The listing builds one solid part. Answer for the finished solid, in the listing's coordinates (mm). Give positions to 0.01 mm unless a question says otherwise; leave off trailing zeros. Write each loop counter-clockwise with the first axis right and the second up, starting at its lowest first coordinate (ties: lowest second). Pieces come first, ordered by that corner, then holes.
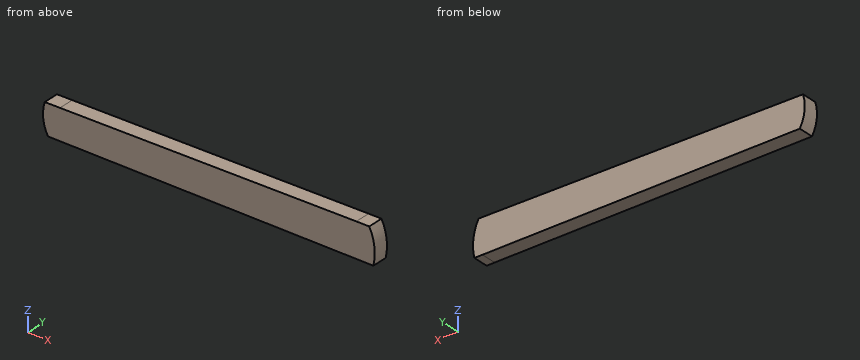
```python
from build123d import *

# Parameters (mm, degrees)
F2_DEPTH = 25


with BuildPart() as f2:
    # F1 (on face) → F2 (new body)
    with BuildSketch(Plane.XZ):
        with BuildLine():
            ThreePointArc((307.522314, 136.204265), (309.150117, 164.161267), (300.922203, 190.929627))
            Line((300.922203, 190.929627), (299.40453, 190.929627))
            Line((299.40453, 190.929627), (280.23421, 190.929627))
            Line((280.23421, 190.929627), (-194.487512, 188.015388))
            Line((-194.487512, 188.015388), (-218.880566, 187.865643))
            ThreePointArc((-218.880566, 187.865643), (-221.348908, 163.277257), (-213.697833, 139.779545))
            Line((-213.697833, 139.779545), (294.608427, 136.292847))
            Line((294.608427, 136.292847), (307.522314, 136.204265))
        make_face()
    extrude(amount=F2_DEPTH)


solid = f2.part
```
Item 1: Each of these flat-tipped pins is pushed along its axis until it touches: P1, Ø1, axis at y = -11, z = 149, coming from the -X side; P2, Ø4, axis at y = -14, z = 167, coming from the -X side; P3, Ø1.5, axis at x = 38.5, y = -3.5, coming from the -Z side. Where does it stop, or does it pass through?
Conclusion:
P1: stops at x = -218.19
P2: stops at x = -221.69
P3: stops at z = 138.04
Item 2: A cutting plane is placed at C-C, the plane x = 96. Give the vertices of the cut face in (y, z), plus the area to 3 significant figures.
Conclusion:
outline: (-25, 137.66) - (0, 137.66) - (0, 189.8) - (-25, 189.8) - close
area: 1,300 mm2
Item 3: A cutting plane is placed at B-B, the plane x = -185. Give the vertices of the cut face in (y, z), plus the area to 3 significant figures.
Conclusion:
outline: (-25, 139.58) - (0, 139.58) - (0, 188.07) - (-25, 188.07) - close
area: 1,210 mm2
Item 4: A cutting plane is placed at A-A, the plane y = -19. Give the vertices of the cut face in (x, z).
Conclusion:
outline: (-218.88, 187.87) arc R60 ccw to (-213.7, 139.78) - (307.52, 136.2) arc R79 ccw to (300.92, 190.93) - (280.23, 190.93) - close
Item 5: Consider probe 1 along X at (y, z) = (-5.5, 174); probe 2 along X at (y, z) = (-16.75, 182); probe 3 along Z at (x, y) = (-138.5, -10.5). Determine where each line is inside the solid, lowest interval first.
Conclusion:
probe 1: x = -221.54 to 307.33
probe 2: x = -220.42 to 304.85
probe 3: z = 139.26 to 188.36
